The model under review builds one solid part; all positions refer to its coordinate system, in mm. Face numbers are marked on the shaded views. Give positions to 0.01 mm unless a question says otherwise; leave off trailing zeros. Order: outer loops, then holes, each group sorted by start corner. A loop starts at its lowest first (then second) coordinate and runs counter-clockwise, first axis right, second up. Notation, with made-up numbers: (31, 45) - (44, 45) arc R29 cw to (44, 79) - close; hole circle Ø3 at (-7, -14). An arc over 180 degrees is marked (long way). Use CSV: the item, a comma, the result in double quotes.
```python
from build123d import *

# Parameters (mm, degrees)
CUT_EXTRUDE_3_DEPTH      = 173.789611956
CUT_EXTRUDE_3_DEPTH_BACK = 173.789611956
SKETCH_2_R               = 10
FILLET_1_R               = 2
CHAMFER_1_SIZE           = 2


with BuildPart() as part:
    # 草图1 → 旋转1 (revolve)
    with BuildSketch(Plane.XY, mode=Mode.PRIVATE) as revolve_1_sk:
        Polygon((0, 0), (10, 0), (10, 70), (32.5, 70), (32.5, 80), (10, 80), (10, 120), (0, 120), align=None)
    revolve(revolve_1_sk.sketch.rotate(Axis((-39.78021978, 0, 0), (1, 0, 0)), 90), axis=Axis((-39.78021978, 0, 0), (1, 0, 0)))

    # 草图2 → 切除-拉伸3 (cut, two sides: drawn at the far end of the back side and taken through both)
    with BuildSketch(Plane(origin=(0, 0, 0), x_dir=(0, 0, -1), z_dir=(1, 0, 0)).offset(-CUT_EXTRUDE_3_DEPTH_BACK)):
        with Locations(Location((100, 0, 0), (0, 0, 180))):
            Circle(SKETCH_2_R)
        with Locations(Location((0, -100, 0), (0, 0, 180))):
            Circle(SKETCH_2_R)
        with Locations(Location((-100, 0, 0), (0, 0, 180))):
            Circle(SKETCH_2_R)
        with Locations(Location((0, 100, 0), (0, 0, 180))):
            Circle(SKETCH_2_R)
    extrude(amount=CUT_EXTRUDE_3_DEPTH + CUT_EXTRUDE_3_DEPTH_BACK, mode=Mode.SUBTRACT)

    # 圆角1
    fillet_1_edges = [part.edges().sort_by_distance(p)[0] for p in [
        (10, 0, -80),
    ]]
    fillet(fillet_1_edges, radius=FILLET_1_R)

    # 倒角1
    chamfer_1_edges = [part.edges().sort_by_distance(p)[0] for p in [
        (0, 0, -120),
        (10, 0, -120),
        (32.5, 0, -80),
        (32.5, 0, -70),
    ]]
    chamfer(chamfer_1_edges, length=CHAMFER_1_SIZE)


solid = part.part
```
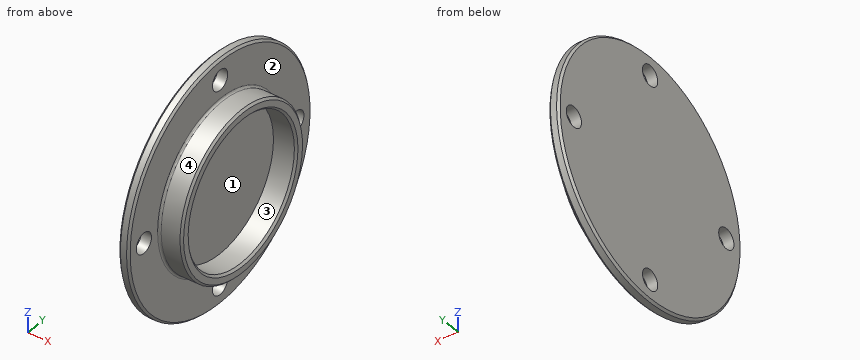
Item 1: Mouldability with a two-part tool opening along Y and no side actions: class the marked faces 1, 2, 3 and 4 as pulls with the +Y half, pulls with the -Y half, needs draft (parallel to the pull), parting line crosses it, or undercut.
Results list:
face 1,"undercut"
face 2,"needs draft"
face 3,"undercut"
face 4,"parting line crosses it"
Item 2: Take a section at A-A, the plane z = 0. State how many separate pieces and enclosed holes the cut face has, and give its area (3 significant figures).
Results list:
separate pieces,"3"
enclosed holes,"0"
area,"2,440 mm2"
Item 3: Wall thickness on L1, parallel to Y at x = 4, z = 0; L2, parallel to Y at x = 23, z = 0; L3, parallel to X at y = 108.5, z = 7.5: over which ranges is each line inside the solid? List them lowest first.
Results list:
L1,"y = -120 to -110, -90 to 90, 110 to 120"
L2,"y = -80 to -70, 70 to 80"
L3,"x = 0 to 10"
Item 4: Clearance check with flat-ended pins moving along their axes: pin 1 (3 mm diameter, centred on y = 57.5, z = 68.5, fed in from -X); pin 2 (10 mm diameter, centred on x = 5, z = -64, fed in from +Y); pin 3 (1 mm diameter, centred on x = 13.5, z = 48.5, fed in from +Y); pin 4 (4 mm diameter, centred on x = 29, y = 4.5, fed in from -Z). State where each tip first meets the part, or that it passes through.
Results list:
pin 1,"stops at x = 0"
pin 2,"stops at y = 104.49"
pin 3,"stops at y = 64"
pin 4,"stops at z = -79.96"
Item 5: Take a section at C-C, the plane x = 27.5. Give the boundary of the cut face in (y, z), and give its area (3 significant figures).
Results list:
outline,"circle Ø160 at (0, 0); hole circle Ø140 at (0, 0)"
area,"4,710 mm2"
